Autodesk Inventor part; units mm, degrees
ref_plane "YZ Plane" through (0, 0, 0) normal (1, 0, 0) x (0, 1, 0)
ref_plane "XZ Plane" through (0, 0, 0) normal (0, 1, 0) x (-1, 0, 0)
ref_plane "XY Plane" through (0, 0, 0) normal (0, 0, 1) x (1, 0, 0)
sketch "Sketch1" plane through (0, 0, 0) normal (0, 1, 0) x (-1, 0, 0)
  line L0 (0, 0) -> (40, 0)
  line L1 (40, 0) -> (40, 52)
  line L2 (40, 52) -> (0, 52)
  line L3 (0, 52) -> (0, 0)
  dimension "d0" = 40
  dimension "d1" = 52
extrude "Extrusion1" add sketch "Sketch1" along normal blind 10.7
sketch "Sketch2" plane through (0, 10.7, 0) normal (0, 1, 0) x (1, 0, 0)
  line L0 (0, 0) -> (-40, 0)
  line L1 (-40, 0) -> (-40, -52)
  line L2 (-40, -52) -> (0, -52)
  line L3 (0, -52) -> (0, 0)
  arc A0 (-23.7, 0) -> (-40, -19.4) centre (-13.6141, -25.0219) ccw
  line L4 (-40, -19.4) -> (0, -19.4) construction
  arc A1 (-40, -30.6438) -> (-13.6141, -52) centre (-13.6141, -25.0219) ccw
  arc A2 (-40, -19.4) -> (-40, -30.6438) centre (-13.6141, -25.0219) ccw
  arc A3 (0, -9.1718) -> (-14.5, 0) centre (-17, -20) ccw
  line L5 (0, -4) -> (-2.8506, -5.6458)
  dimension "d8" = 16.3
  dimension "d9" = 19.4
  dimension "d12" = 20
  dimension "d13" = 17
  dimension "d14" = 14.5
  dimension "d15" = 4
  dimension "d16" = 30
extrude "Extrusion2" cut sketch "Sketch2" against normal through all contours L3 L5 A3 L0 | A0 L1 L0 | A1 L2 L1
sketch "Sketch4" plane through (0, 10.7, 0) normal (0, 1, 0) x (1, 0, 0)
  line L0 (0, -52) -> (0, -4)
  arc A0 (-2.8506, -5.6458) -> (-14.5, 0) centre (-17, -20) ccw
  line L1 (-14.5, 0) -> (-23.7, 0)
  circle A1 centre (-17, -20) radius 16.1
  line L2 (-3, -12.0495) -> (-3, -27.9505)
  point P0 (0, 0)
  dimension "d17" = 32.2
  dimension "d18" = 3
extrude "Extrusion3" cut sketch "Sketch4" against normal blind 5 contours L2 A1 picked at (-14.3987, -21.2686)
sketch "Sketch5" plane through (0, 0, 52) normal (1, 0, 0) x (0, 0, -1)
  line L0 (48, 0) -> (48, 10.7)
  line L1 (0, 10.7) -> (48, 10.7)
  line L2 (0, 0) -> (0, 10.7)
  line L3 (0, 0) -> (48, 0)
  line L4 (46.8, 9.5) -> (46.8, 1.2)
  line L5 (46.8, 1.2) -> (1.2, 1.2)
  line L6 (1.2, 1.2) -> (1.2, 9.5)
  line L7 (1.2, 9.5) -> (46.8, 9.5)
  point P0 (52, 0)
  dimension "d21" = 1.2
extrude "Extrusion4" cut sketch "Sketch5" against normal blind 2 contours L4 L5 L6 L7
sketch "Sketch6" plane through (-14.5, 0, 0) normal (0, 0, -1) x (-1, 0, 0)
  line L0 (0, 10.7) -> (9.2, 10.7)
  line L1 (-11.6494, 0) -> (-14.5, 0)
  line L2 (-11.6494, 10.7) -> (-11.6494, 0)
  line L3 (-14.5, 10.7) -> (-11.6494, 10.7)
  line L4 (-14.5, 0) -> (-14.5, 10.7)
  line L5 (0, 0) -> (-11.6494, 0)
  line L6 (0, 10.7) -> (0, 0)
  line L7 (-11.6494, 10.7) -> (0, 10.7)
  line L8 (-11.6494, 10.7) -> (-11.6494, 0)
  line L9 (0, 3.9) -> (-14.5, 3.9)
  line L10 (0, 5.5) -> (-13.5, 5.5)
  line L11 (-13.5, 5.5) -> (-13.5, 10.7)
  dimension "d24" = 1
  dimension "d25" = 1.6
  dimension "d26" = 3.9
extrude "Extrusion5" add sketch "Sketch6" against normal up to next contours L9 L4 L3 L11 L10 L2 | L2 L10 L6 L9
sketch "Sketch7" plane through (-14.5, 5.5, 0) normal (0, 1, 0) x (1, 0, 0)
  line L0 (0, 0) -> (13.5, 0)
  circle A0 centre (11, -2) radius 1.45
  line L1 (14.5, 0) -> (14.5, -4)
  dimension "d29" = 2.9
  dimension "d30" = 3.5
  dimension "d31" = 2
extrude "Extrusion6" cut sketch "Sketch7" against normal through all
properties part number "Ventilador"
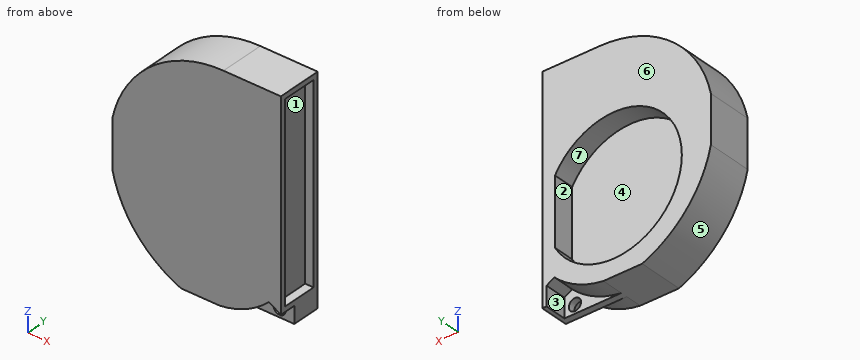
Model file for the job. Use its own axes, mm. Face numbers are marked on the shaded views. A direction names the side the tool comes from. Round coordinates to 2 decimals unless told otherwise and drop trailing zeros. Order: outer loops, then holes, each group sorted by start corner. A loop starts at its lowest first (then second) coordinate and runs counter-clockwise, first axis right, second up. Notation, with made-up numbers: (85, 89.5) -> (142, 89.5) arc R25 ccw to (142, 107.5) -> close; hole circle Ø5 at (82, 40). An arc over 180 degrees is marked (long way). Use one line per item in the form item = value.
Item 1: Cut at D-D, the plane z = 8. Write the cut outline in (x, y), and give its area (3 significant figures).
Returned:
outline = (-34.54, 0) -> (0, 0) -> (0, 1.2) -> (-2, 1.2) -> (-2, 9.5) -> (0, 9.5) -> (0, 10.7) -> (-6.27, 10.7) -> (-6.27, 5.7) -> (-27.73, 5.7) -> (-27.73, 10.7) -> (-34.54, 10.7) -> close
area = 246 mm^2
Item 2: Pull direction X, two halves, no side cores. Call the marked faces 4, 5, 6 and 7: released by +X, released by -X, zero draft, split by the parting line, or undercut.
Returned:
face_4 = undercut
face_5 = released by -X
face_6 = zero draft
face_7 = undercut
Item 3: Cut at A-A, the plane z = 2. Write the cut outline in (x, y).
Returned:
outline = (-27.68, 0) -> (-7.93, 0) -> (-7.93, 3.9) -> (-4.95, 3.9) -> (-4.95, 5.5) -> (-7.93, 5.5) -> (-7.93, 10.7) -> (-27.68, 10.7) -> close; (-2.05, 3.9) -> (0, 3.9) -> (0, 10.7) -> (-1, 10.7) -> (-1, 5.5) -> (-2.05, 5.5) -> close
Item 4: Tool access for the marked faces 1, 2 and 3: list every direction of +Z, -Z, +X, -X, +Y, -Y with a clear straight run to the whole face (end or side of a thin tool).
Returned:
face_1 = +X
face_2 = +Y
face_3 = -Z, +Y
Item 5: Cut at C-C, the plane z = 20. Write the cut outline in (x, y).
Returned:
outline = (-40, 0) -> (0, 0) -> (0, 1.2) -> (-2, 1.2) -> (-2, 9.5) -> (0, 9.5) -> (0, 10.7) -> (-3, 10.7) -> (-3, 5.7) -> (-33.1, 5.7) -> (-33.1, 10.7) -> (-40, 10.7) -> close
Item 6: Cut at B-B, the plane x = -29.5. Write the cut outline in (y, z).
Returned:
outline = (0, 3.22) -> (10.7, 3.22) -> (10.7, 9.85) -> (5.7, 9.85) -> (5.7, 30.15) -> (10.7, 30.15) -> (10.7, 46.83) -> (0, 46.83) -> close
Item 7: Flat gauge pins, fed straight in: pin 1 Ø2.5 at (x, z) = (-3.5, 2) entering from +Y; pin 2 Ø4 at (x, y) = (-32, 8) entering from -Z; pin 3 Ø4 at (y, z) = (4, 24.5) entering from +X; pin 4 Ø1.5 at (x, y) = (-24.5, 7.5) entering from +Z. Where does each tip first touch, or does it go through?
Returned:
pin_1 = through
pin_2 = 3.59
pin_3 = -2
pin_4 = 50.02
Item 8: Drill centre lines: line 1 (X direction, y = 7.4, z = 20); line 2 (Y direction, x = -18, z = 8.5); line 3 (Y direction, x = -1.5, z = 27). Where is each one in solid material? Low to high.
Returned:
line_1 = -40 to -33.1, -3 to -2
line_2 = 0 to 5.7
line_3 = 0 to 1.2, 9.5 to 10.7
